Read the model definition and answer for the solid it produces. Units are mm, in the model's axes. Face numbers are marked on the shaded views. Give positions to 0.01 mm unless a question says otherwise; leave off trailing zeros. Write each loop counter-clockwise with the first axis right and the second up, starting at its lowest first coordinate (ties: lowest second). Pieces come first, ordered by that corner, then holes. Notation, with made-up numbers: M 57.5,12 L 100.5,12 A12 cw 100.5,17 Z; hole C 14,22.5 d1. An arc over 180 degrees is marked long. Use a Markdown table: item, result. Add a question column.
Item 1: A cutting plane is placed at C-C on z = 0. Determine the outline of the cut face in (x, y), then the cut area to 3 significant figures.
Item 2: The mould has two halves that part along X. Classify the marked faces 1 and 2: pulls with the +X half, pulls with the -X half, needs draft (parallel to the pull), parting line crosses it, or undercut.
Item 3: Consider probe 1 along X at (y, z) = (3, -15.5); probe 2 along X at (y, z) = (2, -22); probe 3 along Y at (x, z) = (17, -19.5). Determine where each line is inside the solid, lowest interval first. Write a range as [from, to].
Item 4: A cutting plane is placed at D-D on x = -47. Determine the outline of the cut face in (y, z), then the cut area to 3 significant figures.
Item 5: A cutting plane is placed at A-A on x = 0. Determine the outline of the cut face in (y, z).
Item 6: A cutting plane is placed at B-B on z = -20. Determine the outline of the cut face in (x, y), then the cut area to 3 significant figures.
Item 7: Given P1, Ø3, axis at y = 1.5, z = 24.5, coming from the -X side; P2, Ø4, axis at y = 1, z = -41.5, coming from the +X side; P3, Ø7, axis at x = 34.64, z = 20, coming from the +Y side, each flat-ended and moving along its own axis, determine where each tip first touches the part or whether it passes through.
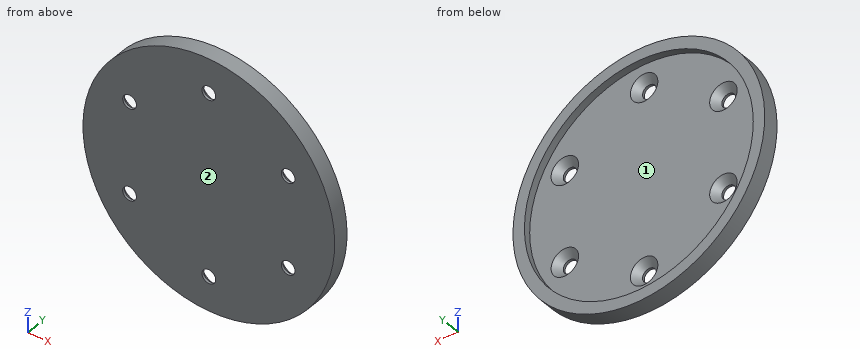
from build123d import *

# Parameters (mm, degrees)
SKETCH2_R          = 3
CUT_EXTRUDE1_DEPTH = 78.884529914
CHAMFER1_SIZE      = 3


with BuildPart() as part:
    # Sketch1 → Revolve1 (revolve)
    with BuildSketch(Plane.XY, mode=Mode.PRIVATE) as revolve1_sk:
        Polygon((50, 3.478641915), (50, 6.478641915), (55, 6.478641915), (55, -0.521358085), (0, -0.521358085), (0, 3.478641915), align=None)
    revolve(revolve1_sk.sketch.rotate(Axis((0, 0, 0), (0, 1, 0)), 90), axis=Axis((0, 0, 0), (0, 1, 0)))

    # Sketch2 → Cut-Extrude1 (cut, through all)
    with BuildSketch(Plane(origin=(0, 3.478641915, 0), x_dir=(1, 0, 0), z_dir=(0, 1, 0))):
        with Locations(Location((0, 40, 0), (0, 0, 270))):
            Circle(SKETCH2_R)
        with Locations(Location((34.641016151, 20, 0), (0, 0, 270))):
            Circle(SKETCH2_R)
        with Locations(Location((34.641016151, -20, 0), (0, 0, 270))):
            Circle(SKETCH2_R)
        with Locations(Location((0, -40, 0), (0, 0, 270))):
            Circle(SKETCH2_R)
        with Locations(Location((-34.641016151, -20, 0), (0, 0, 270))):
            Circle(SKETCH2_R)
        with Locations(Location((-34.641016151, 20, 0), (0, 0, 270))):
            Circle(SKETCH2_R)
    extrude(amount=-CUT_EXTRUDE1_DEPTH, mode=Mode.SUBTRACT)

    # Chamfer1
    chamfer1_edges = [part.edges().sort_by_distance(p)[0] for p in [
        (0, 3.478641915, -43),
        (-34.641016151, 3.478641915, -23),
        (-34.641016151, 3.478641915, 17),
        (0, 3.478641915, 37),
        (34.641016151, 3.478641915, 17),
        (34.641016151, 3.478641915, -23),
    ]]
    chamfer(chamfer1_edges, length=CHAMFER1_SIZE)


solid = part.part
Filled in:
| question | item | result |
|---|---|---|
| 1 | outline | M -55,-0.52 L 55,-0.52 L 55,6.48 L 50,6.48 L 50,3.48 L -50,3.48 L -50,6.48 L -55,6.48 Z |
| 1 | area | 470 mm² |
| 2 | face 1 | undercut |
| 2 | face 2 | needs draft |
| 3 | probe 1 | [-52.77, -37.84], [-31.44, 31.44], [37.84, 52.77] |
| 3 | probe 2 | [-50.41, -38.7], [-30.59, 30.59], [38.7, 50.41] |
| 3 | probe 3 | [-0.52, 3.48] |
| 4 | outline | M -0.52,-28.57 L 6.48,-28.57 L 6.48,-17.06 L 3.48,-17.06 L 3.48,17.06 L 6.48,17.06 L 6.48,28.57 L -0.52,28.57 Z |
| 4 | area | 298 mm² |
| 5 | outline | M -0.52,-55 L 6.48,-55 L 6.48,-50 L 3.48,-50 L 3.48,-46 L 0.48,-43 L -0.52,-43 Z; M -0.52,-37 L 0.48,-37 L 3.48,-34 L 3.48,34 L 0.48,37 L -0.52,37 Z; M -0.52,43 L 0.48,43 L 3.48,46 L 3.48,50 L 6.48,50 L 6.48,55 L -0.52,55 Z |
| 6 | outline | M -51.23,-0.52 L -37.64,-0.52 L -37.64,0.48 L -40.64,3.48 L -45.83,3.48 L -45.83,6.48 L -51.23,6.48 Z; M -31.64,-0.52 L 31.64,-0.52 L 31.64,0.48 L 28.64,3.48 L -28.64,3.48 L -31.64,0.48 Z; M 37.64,-0.52 L 51.23,-0.52 L 51.23,6.48 L 45.83,6.48 L 45.83,3.48 L 40.64,3.48 L 37.64,0.48 Z |
| 6 | area | 376 mm² |
| 7 | P1 | x = -49.96 |
| 7 | P2 | x = 38.27 |
| 7 | P3 | y = 0.98 |
